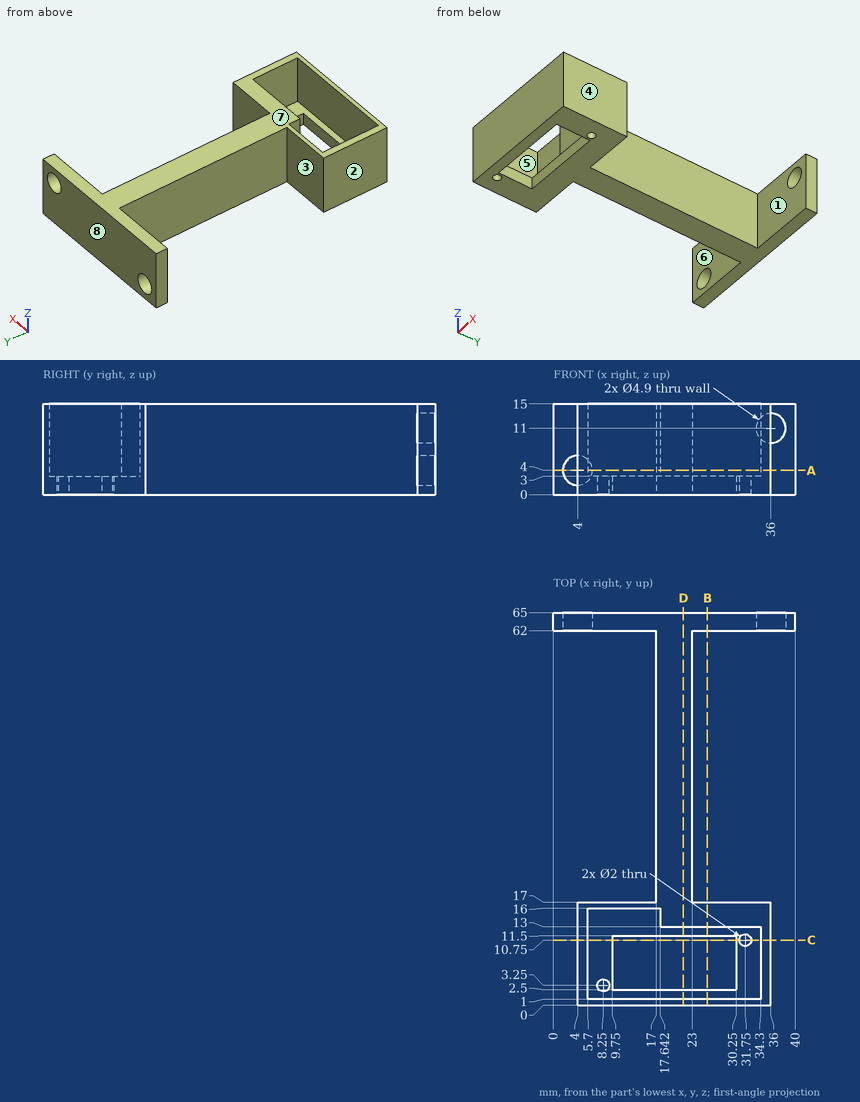
Can you work these out from the drawing? Everything is in mm from the part's minimum corner. A direction names the side the tool comes from. Round coordinates to 2 decimals unless told otherwise and drop trailing zeros. Order: outer loops, then holes, each group sorted by start corner. A loop starts at its lowest first (then second) coordinate and runs counter-clockwise, first axis right, second up.
(1) We'd pull the mould along Y, two halves only. Please class the marked faces 6, 7 and 8: +Y half, -Y half, draft (parallel to the pull), parting line (faces both ways), or undercut.
Results are:
face 6: undercut
face 7: draft
face 8: +Y half
(2) If we section it at D-D (x = 21.5): Please give me the cut outline in (y, z).
Results are:
outline: (0, 0) - (2.5, 0) - (2.5, 3) - (1, 3) - (1, 15) - (0, 15) - close; (11.5, 0) - (65, 0) - (65, 15) - (13, 15) - (13, 3) - (11.5, 3) - close
(3) If we section it at A-A (z = 4): Please give me the cut outline in (x, y).
Results are:
outline: (0, 62) - (1.55, 62) - (1.55, 65) - (0, 65) - close; (4, 0) - (36, 0) - (36, 17) - (23, 17) - (23, 62) - (40, 62) - (40, 65) - (6.45, 65) - (6.45, 62) - (17, 62) - (17, 17) - (4, 17) - close; hole (5.7, 1) - (34.3, 1) - (34.3, 13) - (17.64, 13) - (17.64, 16) - (5.7, 16) - close
(4) If I drill on L1, parallel to Y at x = 9, z = 13.5; L2, parallel to X at y = 3.25, z = 1.6; L3, parallel to Y at x = 34, z = 13.75, over which ranges is the centre line in solid material (lowest first)?
Results are:
L1: y = 0 to 1, 16 to 17, 62 to 65
L2: x = 4 to 7.25, 9.25 to 9.75, 30.25 to 36
L3: y = 0 to 1, 13 to 17, 62 to 65
(5) I'm going to push flat-ended pins straight in: pin 1 (2 mm diameter, centred on x = 12.5, z = 6.5, fed in from -Y); pin 2 (7.5 mm diameter, centred on y = 28.5, z = 6, fed in from -X); pin 3 (1.2 mm diameter, centred on x = 8.25, y = 3.25, fed in from -Z); pin 4 (0.9 mm diameter, centred on y = 14.5, z = 8.5, fed in from -X). Where does each tip first touch, or does it pass through?
Results are:
pin 1: stops at y = 0
pin 2: stops at x = 17
pin 3: passes through
pin 4: stops at x = 4
(6) If we section it at C-C (y = 10.75): Please give me the cut outline in (x, z), plus the area to 3 significant figures.
Results are:
outline: (4, 0) - (9.75, 0) - (9.75, 3) - (5.7, 3) - (5.7, 15) - (4, 15) - close; (30.25, 0) - (30.75, 0) - (30.75, 3) - (30.25, 3) - close; (32.75, 0) - (36, 0) - (36, 15) - (34.3, 15) - (34.3, 3) - (32.75, 3) - close
area: 69.3 mm2
(7) If we section it at B-B (x = 25.5): Please give me the cut outline in (y, z), plus the area to 3 significant figures.
Results are:
outline: (0, 0) - (2.5, 0) - (2.5, 3) - (1, 3) - (1, 15) - (0, 15) - close; (11.5, 0) - (17, 0) - (17, 15) - (13, 15) - (13, 3) - (11.5, 3) - close; (62, 0) - (65, 0) - (65, 15) - (62, 15) - close
area: 129 mm2
(8) On a 3-axis mill with a long thin cutter (end or side, diameter ignored), from which of +Z, -Z, +X, -X, +Y, -Y can I reach the whole of each face in a straight line? I mean the marked faces 1, 2, 3, 4 and 5. Say none if no direction works.
Results are:
face 1: +Z, -Z, +X
face 2: +Z, -Z, -X, -Y
face 3: +Z, -Z, -X
face 4: +Z, -Z, +X, -Y
face 5: +Z
